from build123d import *

# Parameters (mm, degrees)
SKETCH1_W           = 135
SKETCH1_H           = 20
BOSS_EXTRUDE1_DEPTH = 5.4
CHAMFER1_SIZE       = 2
SKETCH2_W           = 131
SKETCH2_H           = 4
BOSS_EXTRUDE2_DEPTH = 5


with BuildPart() as part:
    # Sketch1 → Boss-Extrude1 (new body)
    with BuildSketch(Plane(origin=(0, 0, 0), x_dir=(1, 0, 0), z_dir=(0, 1, 0))):
        Rectangle(SKETCH1_W, SKETCH1_H)
    extrude(amount=BOSS_EXTRUDE1_DEPTH)

    # Chamfer1
    chamfer1_edges = [part.edges().sort_by_distance(p)[0] for p in [
        (-67.5, 5.4, 0),
        (0, 5.4, 10),
        (67.5, 5.4, 0),
        (0, 5.4, -10),
    ]]
    chamfer(chamfer1_edges, length=CHAMFER1_SIZE)

    # Sketch2 → Boss-Extrude2 (add)
    with BuildSketch(Plane(origin=(0, 5.4, 0), x_dir=(1, 0, 0), z_dir=(0, 1, 0))):
        with Locations((0, 6)):
            Rectangle(SKETCH2_W, SKETCH2_H)
        with Locations((0, -6)):
            Rectangle(SKETCH2_W, SKETCH2_H)
    extrude(amount=BOSS_EXTRUDE2_DEPTH)


solid = part.part
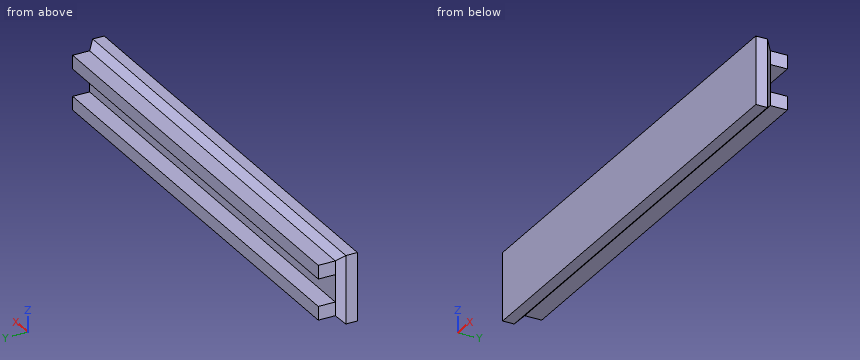
CAD build for the part. Positions are in the model's coordinates, mm. Round coordinates to 2 decimals unless told otherwise and drop trailing zeros. Write each loop counter-clockwise with the first axis right and the second up, starting at its lowest first coordinate (ties: lowest second). Pieces come first, ordered by that corner, then holes. Notation, with made-up numbers: (-30, 62) -> (-5, 62) arc R34 cw to (-5, 99) -> close; hole circle Ø8 at (74.5, -29.75). An arc over 180 degrees is marked (long way). Answer as a JSON object with one key per item and string values.
(1) Band-saw the part on B-B, the plane z = 5.5. List the corners of the cut face in (x, y), then the cut area to 3 significant figures.
Reported:
{"outline": "(-67.5, 0) -> (67.5, 0) -> (67.5, 3.4) -> (65.5, 5.4) -> (65.5, 10.4) -> (-65.5, 10.4) -> (-65.5, 5.4) -> (-67.5, 3.4) -> close", "area": "1,380 mm^2"}
(2) Band-saw the part on D-D, the plane z = -1. List the corners of the cut face in (x, y).
Reported:
{"outline": "(-67.5, 0) -> (67.5, 0) -> (67.5, 3.4) -> (65.5, 5.4) -> (-65.5, 5.4) -> (-67.5, 3.4) -> close"}
(3) Band-saw the part on C-C, the plane x = -56.5. List the corners of the cut face in (y, z).
Reported:
{"outline": "(0, -10) -> (3.4, -10) -> (5.4, -8) -> (10.4, -8) -> (10.4, -4) -> (5.4, -4) -> (5.4, 4) -> (10.4, 4) -> (10.4, 8) -> (5.4, 8) -> (3.4, 10) -> (0, 10) -> close"}
(4) Pin check, flat tips, straight feed: P1, Ø4, axis at x = 0.5, y = 6.5, coming from the -Z side; P2, Ø4.5, axis at y = 8.5, z = -6.5, coming from the +X side; P3, Ø9, axis at x = 25.5, z = -2, coming from the +Y side; P4, Ø6, axis at x = 44.5, y = 8, coming from the +Z side. Stop position of each tip, or through.
Reported:
{"P1": "stops at z = -8.9", "P2": "stops at x = 65.5", "P3": "stops at y = 10.4", "P4": "stops at z = 8.4"}
(5) Band-saw the part on A-A, the plane y = 6.5. List the corners of the cut face in (x, z).
Reported:
{"outline": "(-65.5, -8) -> (65.5, -8) -> (65.5, -4) -> (-65.5, -4) -> close; (-65.5, 4) -> (65.5, 4) -> (65.5, 8) -> (-65.5, 8) -> close"}
(6) Probe probe 1 along Z at (x, y) = (-53, 9.25); probe 2 along Y at (x, z) = (-24.5, -0.25); probe 3 along Y at (x, z) = (0.5, -9). List the from-to ranges inside material, lowest first. Write a range as [from, to].
Reported:
{"probe 1": "z = [-8, -4], [4, 8]", "probe 2": "y = [0, 5.4]", "probe 3": "y = [0, 4.4]"}
